```python
from build123d import *

# Parameters (mm, degrees)
SKETCH2_W           = 120.952956328
SKETCH2_H           = 3.175
BOSS_EXTRUDE1_DEPTH = 95.25
SKETCH3_R           = 39.37
CUT_EXTRUDE2_DEPTH  = 4.175
CUT_EXTRUDE3_DEPTH  = 4.175
SKETCH8_R           = 1.75
CUT_EXTRUDE7_DEPTH  = 4.175
SKETCH10_R          = 1.75
CUT_EXTRUDE9_DEPTH  = 4.175
SKETCH11_W          = 6.35
SKETCH11_H          = 95.25
CUT_EXTRUDE10_DEPTH = 4.175
SKETCH12_R          = 1.75
CUT_EXTRUDE11_DEPTH = 4.175


with BuildPart() as part:
    # Sketch2 → Boss-Extrude1 (new body)
    with BuildSketch(Plane.XY):
        with Locations((98.782063621, 1.5875)):
            Rectangle(SKETCH2_W, SKETCH2_H)
    extrude(amount=BOSS_EXTRUDE1_DEPTH)

    # Sketch3 → Cut-Extrude2 (cut, through all)
    with BuildSketch(Plane(origin=(0, 3.175, 0), x_dir=(1, 0, 0), z_dir=(0, 1, 0))):
        with Locations((111.633541785, -47.625)):
            Circle(SKETCH3_R)
    extrude(amount=-CUT_EXTRUDE2_DEPTH, mode=Mode.SUBTRACT)

    # Sketch4 → Cut-Extrude3 (cut, through all)
    with BuildSketch(Plane(origin=(0, 3.175, 0), x_dir=(1, 0, 0), z_dir=(0, 1, 0))):
        with BuildLine():
            Line((111.633541785, -95.25), (179.051442703, -95.25))
            Line((179.051442703, -95.25), (179.051442703, 0))
            Line((179.051442703, 0), (111.633541785, 0))
            ThreePointArc((111.633541785, 0), (159.258541785, -47.625), (111.633541785, -95.25))
        make_face()
    extrude(amount=-CUT_EXTRUDE3_DEPTH, mode=Mode.SUBTRACT)

    # Sketch8 → Cut-Extrude7 (cut, through all)
    with BuildSketch(Plane(origin=(0, 3.175, 0), x_dir=(1, 0, 0), z_dir=(0, 1, 0))):
        with Locations((76.708541785, -12.7)):
            Circle(SKETCH8_R)
        with Locations((76.708541785, -82.55)):
            Circle(SKETCH8_R)
    extrude(amount=-CUT_EXTRUDE7_DEPTH, mode=Mode.SUBTRACT)

    # Sketch10 → Cut-Extrude9 (cut, through all)
    with BuildSketch(Plane(origin=(0, 3.175, 0), x_dir=(1, 0, 0), z_dir=(0, 1, 0))):
        with Locations((133.541041785, -9.680096933)):
            Circle(SKETCH10_R)
    extrude(amount=-CUT_EXTRUDE9_DEPTH, mode=Mode.SUBTRACT)

    # Sketch11 → Cut-Extrude10 (cut, through all)
    with BuildSketch(Plane(origin=(0, 3.175, 0), x_dir=(1, 0, 0), z_dir=(0, 1, 0))):
        with Locations((41.480585457, -47.625)):
            Rectangle(SKETCH11_W, SKETCH11_H)
    extrude(amount=-CUT_EXTRUDE10_DEPTH, mode=Mode.SUBTRACT)

    # Sketch12 → Cut-Extrude11 (cut, through all)
    with BuildSketch(Plane(origin=(0, 3.175, 0), x_dir=(1, 0, 0), z_dir=(0, 1, 0))):
        with Locations((57.355585457, -69.85)):
            Circle(SKETCH12_R)
    extrude(amount=-CUT_EXTRUDE11_DEPTH, mode=Mode.SUBTRACT)


solid = part.part
```
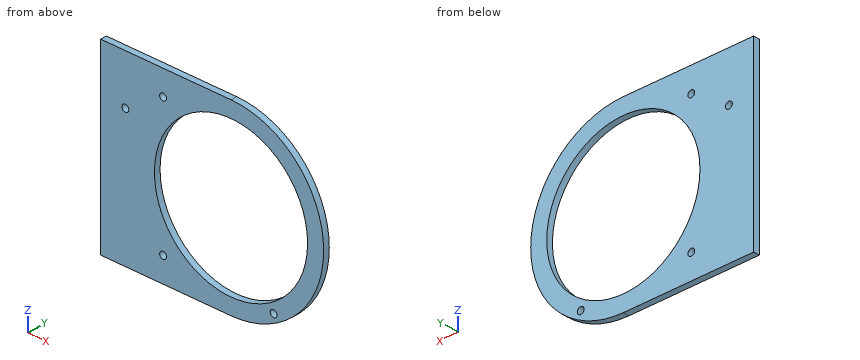
Build history of the part. All positions in model axes, mm. Round coordinates to 2 decimals unless told otherwise and drop trailing zeros. Write each loop counter-clockwise with the first axis right and the second up, starting at its lowest first coordinate (ties: lowest second). Pieces come first, ordered by that corner, then holes. Notation, with made-up numbers: (88.25, -32) - (102.25, -32) arc R12 cw to (102.25, -20) - close; hole circle Ø9 at (77, 17). An arc over 180 degrees is marked (long way). Write each question's results on one line, items separated by ' | '. Start each with the question number.
Item 1: Wall check: L1, parallel to X at y = 2.3, z = 82.55; L2, parallel to Z at x = 110.5, y = 2.7; L3, parallel to X at y = 1.4, z = 81.5. Give the ranges that are in metal, low to high. Write a range as [from, to].
Item 2: Drop a flat-ended pin along its axis: P1, Ø1.5, axis at y = 1.5, z = 80.5, coming from the +X side. Give the stop position or say it passes through.
Item 3: Saw through at A-A (z = 69.85). Write the cut outline in (x, y) (3 decimals), and give its area (3 significant figures).
Item 4: Saw through at D-D (y = 1.6). Write the cut outline in (x, z) (3 decimals).
Item 5: Saw through at B-B (x = 122). Write the cut outline in (y, z) (3 decimals), and give its area (3 significant figures).
Item 6: Saw through at C-C (z = 29.5). Write the cut outline in (x, y) (3 decimals).
Results are:
1) L1: x = [44.66, 74.96], [78.46, 93.46], [129.81, 144.01] | L2: z = [0, 8.27], [86.98, 95.25] | L3: x = [44.66, 75.31], [78.11, 91.57], [131.7, 145.11]
2) P1: stops at x = 146.79
3) outline: (44.656, 0) - (55.606, 0) - (55.606, 3.175) - (44.656, 3.175) - close; (59.106, 0) - (79.137, 0) - (79.137, 3.175) - (59.106, 3.175) - close; (144.13, 0) - (153.755, 0) - (153.755, 3.175) - (144.13, 3.175) - close | area: 129 mm²
4) outline: (44.656, 0) - (111.634, 0) arc R47.625 ccw to (111.634, 95.25) - (44.656, 95.25) - close; hole circle Ø3.5 at (57.356, 69.85); hole circle Ø78.74 at (111.634, 47.625); hole circle Ø3.5 at (76.709, 12.7); hole circle Ø3.5 at (76.709, 82.55); hole circle Ø3.5 at (133.541, 9.68)
5) outline: (0, 1.142) - (3.175, 1.142) - (3.175, 9.644) - (0, 9.644) - close; (0, 85.606) - (3.175, 85.606) - (3.175, 94.108) - (0, 94.108) - close | area: 54.0 mm²
6) outline: (44.656, 0) - (76.684, 0) - (76.684, 3.175) - (44.656, 3.175) - close; (146.583, 0) - (155.675, 0) - (155.675, 3.175) - (146.583, 3.175) - close
